Build history of the part. All positions in model axes, mm. A direction names the side the tool comes from. Round coordinates to 2 decimals unless told otherwise and drop trailing zeros. Write each loop counter-clockwise with the first axis right and the second up, starting at its lowest first coordinate (ties: lowest second). Pieces come first, ordered by that corner, then holes.
Autodesk Inventor part; units mm, degrees
ref_plane "YZ Plane" through (0, 0, 0) normal (1, 0, 0) x (0, 1, 0)
ref_plane "XZ Plane" through (0, 0, 0) normal (0, 1, 0) x (-1, 0, 0)
ref_plane "XY Plane" through (0, 0, 0) normal (0, 0, 1) x (1, 0, 0)
sketch "Sketch1" plane through (0, 0, 0) normal (0, 1, 0) x (-1, 0, 0)
  line L0 (0, -21.0136) -> (0, 21.0817)
  line L1 (-21, 0) -> (21, 0)
  line L2 (21, 0) -> (-21, 0)
  line L3 (0, -21.0136) -> (0, 21.0817)
  line L4 (3.6865, 5.4825) -> (-4.0965, 5.4825)
  line L5 (-5.4825, 3.7546) -> (-5.4825, -4.0284)
  line L6 (-4.0967, -5.4144) -> (3.6863, -5.4144)
  line L7 (5.4825, -4.0284) -> (5.4825, 3.7546)
  line L8 (-5.4825, 5.4825) -> (5.4825, -5.4825) construction
  line L9 (15, 15.0681) -> (15, 4.2181)
  line L10 (15, 4.2181) -> (12.75, 4.2181)
  line L11 (15, 15.0681) -> (4.15, 15.0681)
  line L12 (4.15, 15.0681) -> (4.15, 12.8181)
  line L13 (-15, 14.795) -> (-4.15, 14.795)
  line L14 (-4.15, 14.795) -> (-4.15, 12.75)
  line L15 (-15, 12.75) -> (-15, 14.795)
  line L16 (-15, 14.795) -> (-12.75, 14.795)
  line L17 (-12.75, 3.945) -> (-15, 3.945)
  line L18 (-15, 3.945) -> (-15, 14.795)
  line L19 (-15, -14.9319) -> (-12.75, -14.9319)
  line L20 (-12.75, -4.0819) -> (-15, -4.0819)
  line L21 (-15, -4.0819) -> (-15, -14.9319)
  line L22 (-15, -14.9319) -> (-4.1502, -14.9319)
  line L23 (-4.1502, -14.9319) -> (-4.1502, -12.6819)
  line L24 (-15, -12.7481) -> (-15, -14.9319)
  line L25 (15, -14.9319) -> (12.75, -14.9319)
  line L26 (12.75, -4.0819) -> (15, -4.0819)
  line L27 (15, -4.0819) -> (15, -14.9319)
  line L28 (15, -14.9319) -> (4.1502, -14.9319)
  line L29 (4.1502, -14.9319) -> (4.1502, -12.6819)
  line L30 (15, -12.7481) -> (15, -14.9319)
  circle A0 centre (0, 0) radius 3.1425
  line L31 (8.9925, -14.9319) -> (4.1502, -14.9319)
  line L32 (-4.1502, -14.9319) -> (-8.9925, -14.9319)
  line L33 (15, -14.9319) -> (4.1502, -14.9319)
  line L34 (-4.1502, -14.9319) -> (-15, -14.9319)
  line L35 (15, -8.9925) -> (15, -4.0819)
  line L36 (15, 4.2181) -> (15, 9.0606)
  line L37 (15, 15.0681) -> (15, 4.2181)
  line L38 (15, -4.0819) -> (15, -14.9319)
  line L39 (-8.9925, 14.795) -> (-4.15, 14.795)
  line L40 (4.15, 15.0681) -> (8.9925, 15.0681)
  line L41 (-15, 14.795) -> (-4.15, 14.795)
  line L42 (4.15, 15.0681) -> (15, 15.0681)
  line L43 (-15, 8.9925) -> (-15, 3.945)
  line L44 (-15, -4.0819) -> (-15, -8.9925)
  line L45 (-15, -14.9319) -> (-15, -4.0819)
  line L46 (-15, 3.945) -> (-15, 14.795)
  line L47 (-4.1502, -12.6819) -> (-9.1977, -12.6819)
  line L48 (-12.75, -9.1294) -> (-12.75, -4.0819)
  line L49 (-12.75, -9.1294) -> (-10.5835, -9.1294)
  line L50 (-9.1977, -12.6819) -> (-9.1977, -10.5154)
  line L51 (-9.1975, 10.5835) -> (-9.1975, 12.75)
  line L52 (4.15, 12.8181) -> (8.7875, 12.8181)
  line L53 (12.75, 4.2181) -> (12.75, 8.8556)
  line L54 (12.75, 8.8556) -> (10.5835, 8.8556)
  line L55 (8.7875, 12.8181) -> (8.7875, 10.5835)
  line L56 (4.1502, -12.6819) -> (8.7873, -12.6819)
  line L57 (14.341, -12.7481) -> (15, -12.7481)
  line L58 (12.75, -14.9319) -> (12.75, -14.2729)
  line L59 (12.75, -9.1294) -> (12.75, -4.0819)
  line L60 (10.5835, -9.1294) -> (12.75, -9.1294)
  line L61 (8.7873, -10.5154) -> (8.7873, -12.6819)
  line L62 (5.4825, 5.4825) -> (-0.7955, -0.7955) construction
  line L63 (-2.2221, -2.2221) -> (-5.4825, -5.4825) construction
  line L64 (-12.75, 14.795) -> (-12.75, 14.136)
  line L65 (-12.75, 8.8556) -> (-12.75, 3.945)
  line L66 (-4.15, 12.75) -> (-9.1975, 12.75)
  line L67 (-14.341, 12.75) -> (-15, 12.75)
  line L68 (-10.5835, 8.8556) -> (-12.75, 8.8556)
  line L69 (-5.4825, 3.7546) -> (-10.5835, 8.8556)
  line L70 (-4.0965, 5.4825) -> (-9.1975, 10.5835)
  line L71 (8.7875, 10.5835) -> (3.6865, 5.4825)
  line L72 (10.5835, 8.8556) -> (5.4825, 3.7546)
  line L73 (10.5835, -9.1294) -> (5.4825, -4.0284)
  line L74 (8.7873, -10.5154) -> (3.6863, -5.4144)
  line L75 (-4.0967, -5.4144) -> (-9.1977, -10.5154)
  line L76 (-5.4825, -4.0284) -> (-10.5835, -9.1294)
  line L77 (15, 15) -> (-15, -15) construction
  line L78 (-15, 15) -> (15, -15) construction
  point P0 (-15, 0)
  dimension "d26" = 6.285
  dimension "d0" = 30
  dimension "d1" = 30
  dimension "d2" = 10.965
  dimension "d3" = 10.965
  dimension "d4" = 30
  dimension "d5" = 17.985
  dimension "d6" = 17.985
  dimension "d11" = 10.85
  dimension "d12" = 2.25
  dimension "d13" = 10.85
  dimension "d14" = 2.25
  dimension "d15" = 10.85
  dimension "d16" = 2.25
  dimension "d17" = 10.85
  dimension "d18" = 2.25
  dimension "d19" = 10.85
  dimension "d20" = 10.85
  dimension "d21" = 2.25
  dimension "d22" = 2.25
  dimension "d23" = 10.85
  dimension "d24" = 10.85
  dimension "d25" = 2.25
  dimension "d31" = 30
  dimension "d32" = 30
extrude "Extrusion1" add sketch "Sketch1" along normal blind 275 contours L6 L75 L50 L47 L23 L22 L19 L21 L20 L48 L49 L76 L5 L1 A0 L0 | L0 A0 L1 L7 L73 L60 L59 L26 L27 L25 L28 L29 L56 L61 L74 L6 | L1 L5 L69 L68 L65 L17 L18 L15 L13 L14 L66 L51 L70 L4 L0 A0 | A0 L0 L4 L71 L55 L52 L12 L11 L9 L10 L53 L54 L72 L7 L1
fillet "Fillet1" radius 0.5 20 edges at (15, 137.5, 14.795) (4.15, 137.5, 14.795) (-4.15, 137.5, 15.0681) (-4.15, 137.5, 12.8181) (15, 137.5, 3.945) (12.75, 137.5, 3.945) (15, 137.5, -4.0819) (12.75, 137.5, -4.0819) (15, 137.5, -14.9319) (4.1502, 137.5, -12.6819) (-4.1502, 137.5, -14.9319) (-4.1502, 137.5, -12.6819) (4.1502, 137.5, -14.9319) (-15, 137.5, -14.9319) (-12.75, 137.5, -4.0819) (-15, 137.5, -4.0819) (-12.75, 137.5, 4.2181) (-15, 137.5, 4.2181) (-15, 137.5, 15.0681) (4.15, 137.5, 12.75)
fillet "Fillet2" radius 0.75 24 edges at (-10.5835, 137.5, 8.8556) (-5.4825, 137.5, 3.7546) (-12.75, 137.5, -9.1294) (-10.5835, 137.5, -9.1294) (-8.7873, 137.5, -12.6819) (5.4825, 137.5, -4.0284) (10.5835, 137.5, -9.1294) (-3.6865, 137.5, 5.4825) (-8.7875, 137.5, 10.5835) (5.4825, 137.5, 3.7546) (10.5835, 137.5, 8.8556) (12.75, 137.5, 8.8556) (12.75, 137.5, -9.1294) (4.0965, 137.5, 5.4825) (9.1975, 137.5, 10.5835) (9.1975, 137.5, 12.75) (-8.7875, 137.5, 12.8181) (-12.75, 137.5, 8.8556) (4.0967, 137.5, -5.4144) (9.1977, 137.5, -10.5154) (9.1977, 137.5, -12.6819) (-8.7873, 137.5, -10.5154) (-3.6863, 137.5, -5.4144) (-5.4825, 137.5, -4.0284)
properties part number "Profile_30mm_275mm"
1) Mould opens along Z. For faces 5 (the flat face through (-5.482, 136, 0)), 6 (the flat face through (-10, 136, 15.068)), 7 (the flat face through (-10, 136, -14.932)) say: released by +Z, released by -Z, zero draft, split by the parting line, or undercut.
Results:
face 5: undercut
face 6: released by +Z
face 7: released by -Z
2) Slice it at A-A (x = 0). Write the cut outline in (y, z).
Results:
outline: (0, -5.41) - (275, -5.41) - (275, -3.14) - (0, -3.14) - close; (0, 3.14) - (275, 3.14) - (275, 5.48) - (0, 5.48) - close
3) Slice it at B-B (z = 0). Write the cut outline in (x, y).
Results:
outline: (-5.48, 0) - (-3.14, 0) - (-3.14, 275) - (-5.48, 275) - close; (3.14, 0) - (5.48, 0) - (5.48, 275) - (3.14, 275) - close
4) Wall check: L1, parallel to Z at x = 0, y = 106; L2, parallel to X at y = 214.5, z = -13; L3, parallel to Z at x = -8.5, y = 42. Give the ranges that are in metal, low to high.
Results:
L1: z = -5.41 to -3.14, 3.14 to 5.48
L2: x = -15 to -4.18, 4.18 to 15
L3: z = -14.93 to -12.52, -10.23 to -7.05, 6.77 to 10.3, 12.66 to 15.07
5) Which spindle directions (+Z, -Z, +X, -X, +Y, -Y) get a long thin tool onto all of the face, cutting with end or side? Do faces 1 (the flat face through (0, 136, 5.482)), 2 (the flat face through (-6.27, 135.575, 8.066)), 3 (the flat face through (10, 136, 14.795)), 4 (the flat face through (5.482, 136, 0)). Say none if no direction does.
Results:
face 1: +Z, +Y, -Y
face 2: +Y, -Y
face 3: +Z, +X, +Y, -Y
face 4: +X, +Y, -Y
6) Pin check, flat tips, straight feed: pin 1 Ø8 at (x, y) = (9, 73) entering from +Z (3 decimals); pin 2 Ø1.5 at (x, z) = (-5.5, 11.5) entering from +Y; pin 3 Ø1.5 at (y, z) = (73, -0.5) entering from -X; pin 4 Ø3.5 at (x, y) = (1.5, 133) entering from +Z. Stop position of each tip, or through.
Results:
pin 1: stops at z = 14.795
pin 2: passes through
pin 3: stops at x = -5.48
pin 4: stops at z = 5.48
